```python
from build123d import *

# Parameters (mm, degrees)
ESQUISSE1_R                  = 5
BOSS_EXTRU_1_DEPTH           = 10
ESQUISSE2_R                  = 2.5
BOSS_EXTRU_2_DEPTH           = 5
ESQUISSE3_R                  = 5
BOSS_EXTRU_4_DEPTH           = 10
ESQUISSE4_R                  = 1.5
ENL_V_MAT_EXTRU_1_DEPTH      = 10
ENL_V_MAT_EXTRU_2_DEPTH      = 10
ENL_V_MAT_EXTRU_2_DEPTH_BACK = 10
ESQUISSE5_R                  = 1


with BuildPart() as part:
    # Esquisse1 → Boss.-Extru.1 (new body)
    with BuildSketch(Plane.XY):
        Circle(ESQUISSE1_R)
    extrude(amount=BOSS_EXTRU_1_DEPTH)

    # Esquisse2 → Boss.-Extru.2 (add)
    with BuildSketch(Plane.XY.offset(10)):
        Circle(ESQUISSE2_R)
    extrude(amount=BOSS_EXTRU_2_DEPTH)

    # Esquisse3 → Boss.-Extru.4 (add)
    with BuildSketch(Plane.XY.offset(15)):
        Circle(ESQUISSE3_R)
    extrude(amount=BOSS_EXTRU_4_DEPTH)

    # Esquisse4 → Enl_v. mat.-Extru.1 (cut)
    with BuildSketch(Plane(origin=(0, 0, 0), x_dir=(-1, 0, 0), z_dir=(0, 0, -1))):
        Circle(ESQUISSE4_R)
    extrude(amount=-ENL_V_MAT_EXTRU_1_DEPTH, mode=Mode.SUBTRACT)

    # Esquisse5 → Enl_v. mat.-Extru.2 (cut, two sides: drawn at the far end of the back side and taken through both)
    with BuildSketch(Plane(origin=(0, 0, 0), x_dir=(1, 0, 0), z_dir=(0, 1, 0)).offset(-ENL_V_MAT_EXTRU_2_DEPTH_BACK)):
        with Locations(Location((0, -5, 0), (0, 0, 270))):
            Circle(ESQUISSE5_R)
    extrude(amount=ENL_V_MAT_EXTRU_2_DEPTH + ENL_V_MAT_EXTRU_2_DEPTH_BACK, mode=Mode.SUBTRACT)


solid = part.part
```
Could you check a few things on this model? Use its own coordinates, in mm. A direction names the side the tool comes from. Coordinates: 2 decimals unless noted, no trailing zeros. Order: outer loops, then holes, each group sorted by start corner. A loop starts at its lowest first (then second) coordinate and runs counter-clockwise, first axis right, second up. Notation, with made-up numbers: M -18,76.25 L 41,76.25 A21 ccw 41,89.25 Z; hole C -1,13.25 d3. An arc over 180 degrees is marked long. Use one line per item in the form item = value. Start each with the question number.
1. Suppose I cut it at C-C on x = 4. Write out the boundary of the cut face in (y, z), then the cut area to 3 significant figures.
2. Please list where these lines run through material, in increasing order: line 1 (Z direction, x = 0, y = 3.6); line 2 (Z direction, x = 4.25, y = -0.5); line 3 (Z direction, x = 0, y = -1.75).
3. We'd pull the mould along Z, two halves only. Please class faces 4 (the flat face through (-1.2, 1.2, 0)), 5 (the cylindrical face through (-1.08, -4.88, 19.93)), 6 (the cylindrical face through (-0.54, -2.44, 12.46)): +Z half, -Z half, draft (parallel to the pull), parting line (faces both ways), or undercut.
4. Suppose I cut it at A-A on x = 0. Write out the boundary of the cut face in (y, z).
5. Suppose I cut it at B-B on y = -3.75. Write out the boundary of the cut face in (x, z), then the cut area to 3 significant figures.
6. On a 3-axis mill with a long thin cutter (end or side, diameter ignored), from which of +Z, -Z, +X, -X, +Y, -Y can I reach the whole of each face in a straight line? I mean faces 1 (the cylindrical face through (0, 3, 6)), 2 (the cylindrical face through (1.5, 0.07, 4.93)), 3 (the flat face through (2, -2, 15)). Say none if no direction works.
7. For pin 1 (3.5 mm diameter, centred on x = 0.5, y = 0.5, fed in from -Z); pin 2 (2.5 mm diameter, centred on x = 0, y = 0, fed in from -Z); pin 3 (3 mm diameter, centred on x = -3.5, z = 9, fed in from +Y); pin 4 (1.2 mm diameter, centred on x = 0, z = 5, fed in from -Y), each with a flat end and sliding along its axis, tell me the tip position at first contact or that it passes through.
8. Suppose I cut it at D-D on z = 4.75. Write out the boundary of the cut face in (x, y), then the cut area to 3 significant figures.
Geometry says:
q1.outline = M -3,0 L 3,0 L 3,10 L -3,10 Z; M -3,15 L 3,15 L 3,25 L -3,25 Z
q1.area = 120 mm^2
q2.line_1 = 0 to 4, 6 to 10, 15 to 25
q2.line_2 = 0 to 10, 15 to 25
q2.line_3 = 0 to 4, 6 to 25
q3.face_4 = -Z half
q3.face_5 = draft
q3.face_6 = undercut
q4.outline = M -5,0 L -1.5,0 L -1.5,4 L -5,4 Z; M -5,6 L -1.5,6 L -1.5,10 L 1.5,10 L 1.5,6 L 5,6 L 5,10 L 2.5,10 L 2.5,15 L 5,15 L 5,25 L -5,25 L -5,15 L -2.5,15 L -2.5,10 L -5,10 Z; M 1.5,0 L 5,0 L 5,4 L 1.5,4 Z
q5.outline = M -3.31,0 L 3.31,0 L 3.31,10 L -3.31,10 Z; M -3.31,15 L 3.31,15 L 3.31,25 L -3.31,25 Z; hole C 0,5 d2
q5.area = 129 mm^2
q6.face_1 = +Y, -Y
q6.face_2 = -Z
q6.face_3 = none
q7.pin_1 = 0
q7.pin_2 = 10
q7.pin_3 = 4.58
q7.pin_4 = through
q8.outline = M -0.97,-4.91 L -0.97,-1.15 A1.5 cw -0.97,1.15 L -0.97,4.91 A5 ccw Z; M 0.97,-4.91 A5 ccw 0.97,4.91 L 0.97,1.15 A1.5 cw 0.97,-1.15 Z
q8.area = 57.6 mm^2
